Geometry check sheet. Reference: the model listing, model coordinates, mm. A direction names the side the tool comes from. Give positions to 0.01 mm unless a question says otherwise; leave off trailing zeros. Loops run counter-clockwise (first coordinate to the right, second up) from the corner with the lowest first, then second, coordinate; pieces in that order, holes last.
1. Cross-section at B-B, the plane z = 0. Record the cut outline in (x, y), plus the area to 3 significant figures.
2. Cross-section at A-A, the plane x = 0. Record the cut outline in (y, z).
3. Material ranges on L1, parallel to X at y = -37, z = 0; L2, parallel to Y at x = -37, z = -15, recorded low to high.
4. Cross-section at D-D, the plane x = -26.5. Record the cut outline in (y, z), plus the area to 3 significant figures.
5. Tool access check on faces 5 (the flat face through (-15.2, -50.8, 5.3)), 6 (the flat face through (24, -25.4, 0)). Record the directions out of +Z, -Z, +X, -X, +Y, -Y that give a thin tool (end or side, any length) a straight path to the whole face; none if there is none.
6. Cross-section at C-C, the plane y = -47. Record the cut outline in (x, z), plus the area to 3 significant figures.
7. Go/stop test with flat-tipped pins: pin 1 Ø8 at (y, z) = (-29.5, -8) entering from +X; pin 2 Ø4 at (x, z) = (10.5, 4) entering from -Y; pin 3 Ø12 at (x, y) = (-9.5, -35.5) entering from +Z. Record where each tip stops, or that it passes through.
8. Release check for a two-part mould opening along X. For faces 1 (the cylindrical face through (20.69, -37.92, -8.58)), 2 (the flat face through (0, -25.4, 0)), 3 (the flat face through (3, 0, 0)), 4 (the cylindrical face through (-3.43, -37.92, -15.43)) record: +X half, -X half, draft (parallel to the pull), parting line (faces both ways), or undercut.
from build123d import *

# Parameters (mm, degrees)
F0_R     = 22.39752
F0_R_2   = 15.804848
F1_DEPTH = 50.8
F2_W     = 95.513668
F2_H     = 67.828547
F3_DEPTH = 25.4


with BuildPart() as f1:
    # F0 (on Front) → F1 (new body)
    with BuildSketch(Plane.XZ):
        Circle(F0_R)
        Circle(F0_R_2, mode=Mode.SUBTRACT)
    extrude(amount=F1_DEPTH)

    # F2 (on Front) → F3 (join)
    with BuildSketch(Plane.XZ):
        with Locations((3.322212, -0.281336)):
            Rectangle(F2_W, F2_H)
    extrude(amount=F3_DEPTH)


solid = f1.part
Result:
1. outline: (-44.43, -25.4) - (-22.4, -25.4) - (-22.4, -50.8) - (-15.8, -50.8) - (-15.8, -25.4) - (15.8, -25.4) - (15.8, -50.8) - (22.4, -50.8) - (22.4, -25.4) - (51.08, -25.4) - (51.08, 0) - (-44.43, 0) - close
1. area: 2,760 mm2
2. outline: (-50.8, -22.4) - (-25.4, -22.4) - (-25.4, -34.2) - (0, -34.2) - (0, 33.63) - (-25.4, 33.63) - (-25.4, 22.4) - (-50.8, 22.4) - (-50.8, 15.8) - (-25.4, 15.8) - (-25.4, -15.8) - (-50.8, -15.8) - close
3. L1: x = -22.4 to -15.8, 15.8 to 22.4
3. L2: y = -25.4 to 0
4. outline: (-25.4, -34.2) - (0, -34.2) - (0, 33.63) - (-25.4, 33.63) - close
4. area: 1,720 mm2
5. face 5: +Z, -Z, +X, -X, -Y
5. face 6: -Y
6. outline: circle Ø44.8 at (0, 0); hole circle Ø31.61 at (0, 0)
6. area: 791 mm2
7. pin 1: stops at x = 22.04
7. pin 2: stops at y = -25.4
7. pin 3: stops at z = 22.12
8. face 1: parting line
8. face 2: undercut
8. face 3: draft
8. face 4: undercut
